Autodesk Fusion 360 part; units mm, degrees
sketch "Sketch1" plane through (0, 0, 0) normal (0, 0, 1) x (1, 0, 0)
  line L0 (9, 3) -> (-9, 3)
  line L1 (-9, 3) -> (-9, -10)
  line L2 (-9, -10) -> (9, -10)
  line L3 (9, -10) -> (9, 3)
  circle A0 centre (-3.5, 0) radius 1.75
  circle A1 centre (-3.5, 0) radius 3
  line L4 (9, -2.8) -> (-9, -2.8)
  line L5 (-9, -2.8) -> (-9, 2.8)
  line L6 (-9, 2.8) -> (9, 2.8)
  line L7 (9, 2.8) -> (9, -2.8)
  line L8 (9, -2.8) -> (-9, 2.8) construction
  line L9 (-9, -2.8) -> (9, 2.8) construction
  dimension "d1" = 18
  dimension "d2" = 13
  dimension "d5" = 3.5
  dimension "d6" = 6
  dimension "d9" = 5.6
  dimension "d12" = 3.5
  dimension "d23" = 3
extrude "Extrude1" add sketch "Sketch1" along normal blind 2
extrude "Extrude2" add sketch "Sketch1" along normal blind 4 contours L0 L3 A1 L6 | L0 L1 A1 L6 | L3 A1 L4 L6 L7 | L1 A1 L4 L5 L6 | L1 L2 L3 A1 L4
extrude "Extrude3" add sketch "Sketch1" against normal blind 1 contours L3 A1 L4 L6 L7 | A1 L4 L6 | L1 A1 L4 L5 L6
sketch "Sketch2" plane through (9, 0, 0) normal (1, 0, 0) x (0, 1, 0)
  line L0 (-10, 0) -> (-2.8, 0)
  line L1 (-2.8, 0) -> (-2.8, -1)
  line L2 (-2.8, -1) -> (2.8, -1)
  line L3 (2.8, -1) -> (2.8, 0)
  line L4 (2.8, 0) -> (3, 0)
  line L5 (3, 0) -> (3, 4)
  line L6 (3, 4) -> (-10, 4)
  line L7 (-10, 4) -> (-10, 0)
  circle A0 centre (-3.5, 5) radius 2.25
  circle A1 centre (-3.5, 5) radius 4.45
  line L8 (-10, 0) -> (3, 0)
  line L9 (-3.5, 4) -> (-3.5, 5) construction
  dimension "d13" = 4.5
  dimension "d14" = 2.2
  dimension "d18" = 5
extrude "Extrude4" cut sketch "Sketch2" against normal blind 3.5 from surface at -3.5 contours L6 A0 A1 picked at (-3.7762, 1.3019)
sketch "Sketch3" plane through (0, 0, 4) normal (0, 0, 1) x (-1, 0, 0)
  line L0 (-2, 5.5156) -> (-5.5, 5.5156)
  line L1 (-5.5, 5.5156) -> (-5.5, 7.8362)
  line L2 (-5.5, 7.8362) -> (-2, 7.8362)
  line L3 (-2, 7.8362) -> (-2, 5.5156)
  line L4 (-5.5, 1.4844) -> (-2, 1.4844)
  line L5 (-2, 1.4844) -> (-2, -0.8362)
  line L6 (-2, -0.8362) -> (-5.5, -0.8362)
  line L7 (-5.5, -0.8362) -> (-5.5, 1.4844)
  line L8 (-9, 10) -> (-9, -3)
  line L9 (-9, -3) -> (3.5, -3)
  circle A0 centre (3.5, 0) radius 3
  line L10 (3.5, -3) -> (9, -3)
  line L11 (9, -3) -> (9, 10)
  line L12 (9, 10) -> (-9, 10)
  line L13 (0.5, 0) -> (0.5, -5.3952)
  arc A1 (0.5, -5.3952) -> (6.5, -5.3952) centre (3.5, -5.3952) ccw
  line L14 (6.5, -5.3952) -> (6.5, 0)
  arc A2 (6.5, 0) -> (0.5, 0) centre (3.5, 0) ccw
  line L15 (3.5, 0) -> (3.5, -5.3952) construction
extrude "Extrude5" cut sketch "Sketch3" against normal up to surface (2 mm away) contours L9 A0 L13 | A0 L10 L14
fillet "Fillet1" radius 2 4 edges at (-9, -10, 2) (9, -10, 2) (9, 3, 2) (-9, 3, 2)
sketch "Sketch4" plane through (0, 0, 2) normal (0, 0, 1) x (-1, 0, 0)
  arc A0 (6.5, 0) -> (0.5, 0) centre (3.5, 0) ccw
  line L0 (0.5, 0) -> (0.5, -3)
  line L1 (0.5, -3) -> (6.5, -3)
  line L2 (6.5, -3) -> (6.5, 0)
  circle A1 centre (3.5, 0) radius 1.75 construction
  line L3 (0.5, -1.75) -> (6.5, -1.75)
  line L4 (5.25, -1.75) -> (5.25, 1.75)
  line L5 (5.9367, 1.75) -> (1.0633, 1.75)
  line L6 (1.75, 1.75) -> (1.75, -1.75)
  line L7 (1.75, -1.75) -> (5.25, 1.75) construction
  line L8 (5.25, -1.75) -> (1.75, 1.75) construction
  point P0 (3.5, 0)
extrude "Extrude6" cut sketch "Sketch4" against normal blind 0.2 contours A0 L2 L3 L4 L5 | A0 L0 L3 L5 L6 | L3 L4 L5 L6
extrude "Extrude7" cut sketch "Sketch4" against normal blind 0.4 contours L3 L4 L5 L6
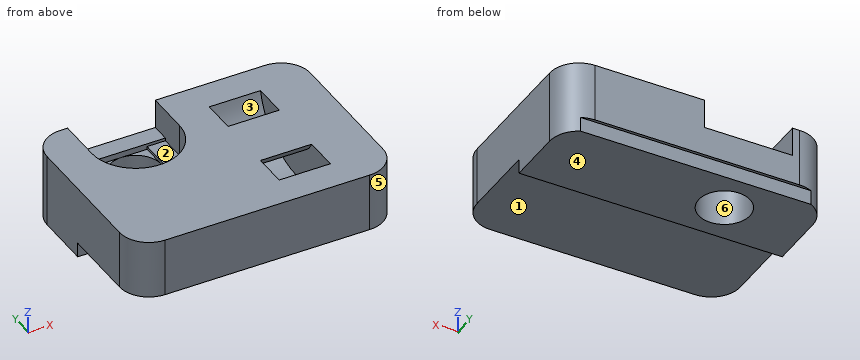
Input: part model. Units: mm. Frame: model coordinates. Face numbers are marked on the shaded views. A direction names the side the tool comes from. Give positions to 0.01 mm unless a question says otherwise; leave off trailing zeros. Write each loop counter-clockwise with the first axis right and the second up, starting at its lowest first coordinate (ties: lowest second). Pieces come first, ordered by that corner, then holes. Notation, with made-up numbers: (28.25, -13.5) - (58.25, -13.5) arc R14 ccw to (58.25, 11.5) - close; hole circle Ø11 at (-39, 19). An arc over 180 degrees is marked (long way). Write item = value, one per line. Start each with the question number.
1. Mould query, pull axis Y, two halves, no side actions, for the marked faces 4, 5 and 6. Classes: released by +Y, released by -Y, zero draft, split by the parting line, or undercut.
2. Section query C-C, the plane y = 1.5. Output: boundary loops of the cut face in (x, z), then the cut area to 3 significant figures.
3. Section query B-B, the plane x = 3.25. Output: boundary loops of the cut face in (y, z).
4. Ray query, L1, parallel to X at y = 0, z = -0.3; L2, parallel to X at y = -6.5, z = 2.35; L3, parallel to Y at x = -4.5, z = 1.75. Return the intervals inside material, ascending.
5. Section query A-A, the plane y = -3.5. Output: boundary loops of the cut face in (x, z).
6. Section query D-D, the plane x = 1.25. Output: boundary loops of the cut face in (y, z), then the cut area to 3 significant figures.
7. Access query for the marked faces 1, 2 and 3. Directions: +Z, -Z, +X, -X, +Y, -Y. A direction counts if a zero-diameter tool reaches every point of the face in a straight line with its end or side. Return the directions, or none.
8. First-contact query: pin 1 Ø0.6 at (x, y) = (-3.5, -2.5) entering from +Z; pin 2 Ø1.1 at (y, z) = (2, 3.5) entering from -X; pin 3 Ø3 at (x, y) = (5, -6) entering from -Z. Flat tips, straight axial feed; report the tip coordinate or a pass-through.
Check sheet entries:
q1.face_4 = zero draft
q1.face_5 = released by -Y
q1.face_6 = undercut
q2.outline = (-8.94, -1) - (-4.4, -1) - (-4.4, 1.6) - (-5.25, 1.6) - (-5.25, 1.8) - (-6.5, 1.8) - (-6.5, 4) - (-8.94, 4) - close; (-2.6, -1) - (8.94, -1) - (8.94, 4) - (-0.5, 4) - (-0.5, 1.8) - (-1.75, 1.8) - (-1.75, 1.6) - (-2.6, 1.6) - close
q2.area = 70.8 mm2
q3.outline = (-10, 0) - (-2.8, 0) - (-2.8, -1) - (2.8, -1) - (2.8, 0) - (3, 0) - (3, 4) - (0.84, 4) arc R4.45 cw to (-7.84, 4) - (-10, 4) - close; (-5.52, 4) arc R2.25 ccw to (-1.48, 4) - close
q4.L1 = -9 to -5.25, -1.75 to 9
q4.L2 = -9 to 2, 5.5 to 9
q4.L3 = -10 to -1.75, 1.75 to 3
q5.outline = (-9, 0) - (9, 0) - (9, 4) - (-9, 4) - close; hole (2, 0.55) - (5.5, 0.55) - (5.5, 2.75) - (2, 2.75) - close
q6.outline = (-10, 0) - (-2.8, 0) - (-2.8, -1) - (2.8, -1) - (2.8, 0) - (3, 0) - (3, 4) - (-10, 4) - close
q6.area = 57.6 mm2
q7.face_1 = -Z, +X, -X, -Y
q7.face_2 = +Z
q7.face_3 = none
q8.pin_1 = 2
q8.pin_2 = -8.95
q8.pin_3 = 0
